Geometry: see drawing. Coordinates: mm, zero at the bounding-box minimum. A direction names the side the tool comes from. Coordinates: 2 decimals unless noted, no trailing zeros. Loops run counter-clockwise (first coordinate to the right, second up) from the corner with the lowest first, then second, coordinate; pieces in that order, holes last. Notation, with made-up numbers: (1.25, 16.25) -> (10.25, 16.25) arc R25 cw to (10.25, 53.25) -> close; hole circle Ø8 at (48.5, -10.75). An arc over 180 degrees is marked (long way). Answer as a JSON object with one key per item and string values.
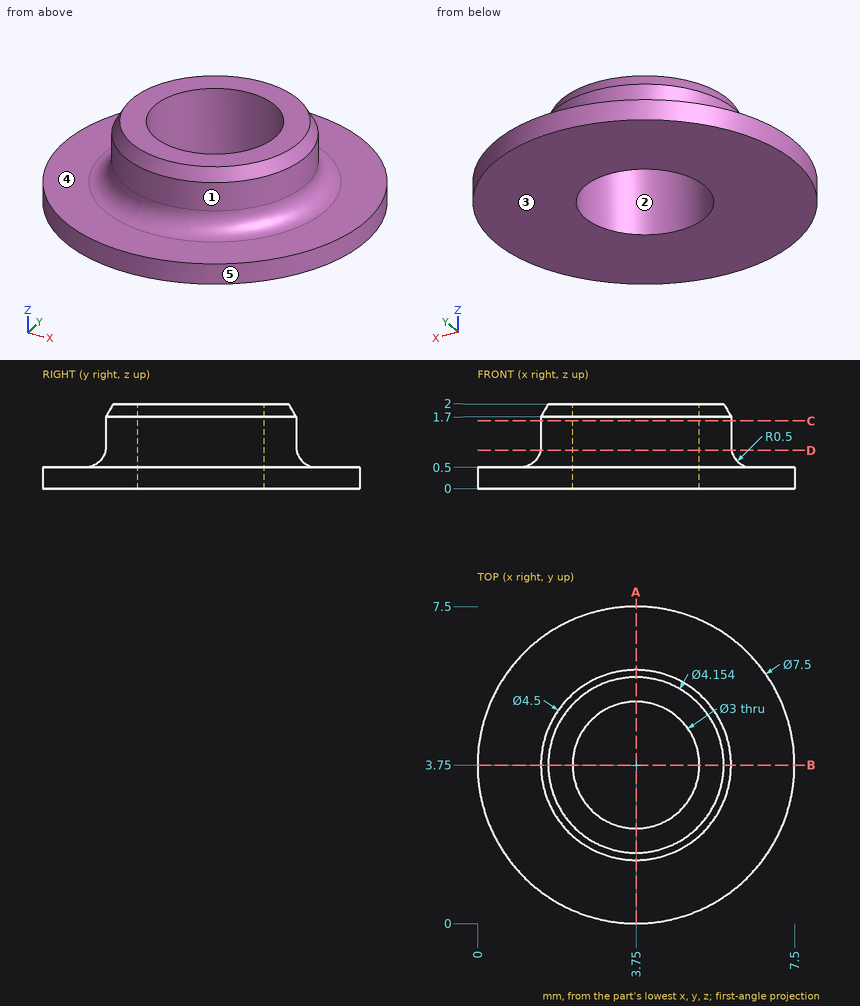
1. Line query: line 1 along Y through (x, z) = (3.75, 0.95); line 2 along Y through (x, z) = (3.75, 0.6). Output: solid intervals per line, ascending.
Reply:
{"line 1": "y = 1.5 to 2.25, 5.25 to 6", "line 2": "y = 1.3 to 2.25, 5.25 to 6.2"}
2. Section query C-C (z = 1.6). Return loops of the section in (x, y).
Reply:
{"outline": "circle Ø4.5 at (3.75, 3.75); hole circle Ø3 at (3.75, 3.75)"}
3. Section query A-A (x = 3.75). Return loops of the section in (y, z).
Reply:
{"outline": "(0, 0) -> (2.25, 0) -> (2.25, 2) -> (1.67, 2) -> (1.5, 1.7) -> (1.5, 1) arc R0.5 cw to (1, 0.5) -> (0, 0.5) -> close; (5.25, 0) -> (7.5, 0) -> (7.5, 0.5) -> (6.5, 0.5) arc R0.5 cw to (6, 1) -> (6, 1.7) -> (5.83, 2) -> (5.25, 2) -> close"}
4. Pin query (flat end, axial travel): P1, Ø1, axis at x = 5, z = 0.5, coming from the -Y side. Return the tip coordinate at first contact, or that it passes through.
Reply:
{"P1": "stops at y = 0.08"}
5. Mould query, pull axis Y, two halves, no side actions, for the marked faces 1, 2 and 3. Classes: pulls with the +Y half, pulls with the -Y half, needs draft (parallel to the pull), parting line crosses it, or undercut.
Reply:
{"face 1": "parting line crosses it", "face 2": "undercut", "face 3": "needs draft"}
6. Section query D-D (z = 0.9). Return loops of the section in (x, y).
Reply:
{"outline": "circle Ø4.52 at (3.75, 3.75); hole circle Ø3 at (3.75, 3.75)"}
7. Access query for the marked faces 4 and 5. Directions: +Z, -Z, +X, -X, +Y, -Y. A direction counts if a zero-diameter tool reaches every point of the face in a straight line with its end or side. Return the directions, or none.
Reply:
{"face 4": "+Z", "face 5": "+Z, -Z"}
